```python
from build123d import *

# Parameters (mm, degrees)
SKETCH_1_R      = 6
EXTRUDE_1_DEPTH = 42.5
EXTRUDE_2_DEPTH = 5


with BuildPart() as part:
    # 草图1 → 凸台-拉伸1 (new body)
    with BuildSketch(Plane(origin=(0, 0, 0), x_dir=(0, 0, -1), z_dir=(1, 0, 0))):
        Circle(SKETCH_1_R)
    extrude(amount=EXTRUDE_1_DEPTH)

    # 草图2 → 凸台-拉伸2 (add)
    with BuildSketch(Plane.ZY):
        Polygon((-5.922430933, 0.537848847), (-5.913562188, -0.627894725), (-5.677438564, -1.769508656), (-5.223134161, -2.843121361), (-4.568107641, -3.807474506), (-3.737531306, -4.625508542), (-2.763323739, -5.265786878), (-1.68292319, -5.703703978), (-0.537848847, -5.922430933), (0.627894725, -5.913562188), (1.769508656, -5.677438564), (2.843121361, -5.223134161), (3.807474506, -4.568107641), (4.625508542, -3.737531306), (5.265786878, -2.763323739), (5.703703978, -1.68292319), (5.922430933, -0.537848847), (5.913562188, 0.627894725), (5.677438564, 1.769508656), (5.223134161, 2.843121361), (4.568107641, 3.807474506), (3.737531306, 4.625508542), (2.763323739, 5.265786878), (1.68292319, 5.703703978), (0.537848847, 5.922430933), (-0.627894725, 5.913562188), (-1.769508656, 5.677438564), (-2.843121361, 5.223134161), (-3.807474506, 4.568107641), (-4.625508542, 3.737531306), (-5.265786878, 2.763323739), (-5.703703978, 1.68292319), align=None)
    extrude(amount=EXTRUDE_2_DEPTH)


solid = part.part
```
Verification items for the finished model (mm, model axes). A direction names the side the tool comes from. Give positions to 0.01 mm unless a question says otherwise; leave off trailing zeros. Loops run counter-clockwise (first coordinate to the right, second up) from the corner with the lowest first, then second, coordinate; pieces in that order, holes last.
1. Section check C-C, the plane x = 6. Enter the section's corners in (y, z).
2. Go/stop test with flat-tipped pins: pin 1 Ø3 at (x, z) = (14, 3.5) entering from +Y; pin 2 Ø4 at (x, z) = (23, -2.5) entering from +Y; pin 3 Ø2 at (x, z) = (14.5, 2) entering from +Y. Record where each tip stops, or that it passes through.
3. Set-up check for faces 1 (the flat face through (-2.46, 3.32, 4.9)), 2 (the flat face through (-2.46, -1.12, 5.81)), 3 (the flat face through (-2.465, -2.299, -5.453)): record each of +Z, -Z, +X, -X, +Y, -Y from which the full face is reachable in a straight line by a thin tool's end or side.
4. Section check A-A, the plane z = -2.25. Enter the section's corners in (x, y).
5. Section check B-B, the plane y = 3.25. Enter the section's corners in (x, z), then the cut area to 3 significant figures.
6. Thickness scan on line 1 (Z direction, x = 24.5, y = -0.25); line 2 (Y direction, x = 37.5, z = -1). Record the ranges inside material, lowest first.
Geometry says:
1. outline: circle Ø12 at (0, 0)
2. pin 1: stops at y = 5.66
2. pin 2: stops at y = 5.98
2. pin 3: stops at y = 5.92
3. face 1: +Z, -X, +Y
3. face 2: +Z, -X, -Y
3. face 3: -Z, -X, -Y
4. outline: (-5, -5.47) - (0, -5.47) - (0, -5.56) - (42.5, -5.56) - (42.5, 5.56) - (0, 5.56) - (0, 5.47) - (-5, 5.47) - close
5. outline: (-5, -4.95) - (0, -4.95) - (0, -5.04) - (42.5, -5.04) - (42.5, 5.04) - (0, 5.04) - (0, 4.95) - (-5, 4.95) - close
5. area: 478 mm2
6. line 1: z = -5.99 to 5.99
6. line 2: y = -5.92 to 5.92
